For this review, take the finished solid that the model builds, in its own axes (mm). A direction names the side the tool comes from. Round coordinates to 2 decimals unless told otherwise and drop trailing zeros. Loops run counter-clockwise (first coordinate to the right, second up) from the corner with the lowest first, then second, coordinate; pieces in that order, holes last. Notation, with made-up numbers: (19, 29.25) -> (51, 29.25) arc R19 ccw to (51, 44.25) -> close; hole circle Ø3 at (65, -24). An arc over 180 degrees is marked (long way). Write each question's results on one line, items separated by ' | '.
```python
from build123d import *

# Parameters (mm, degrees)
SKETCH1_W           = 48
SKETCH1_H           = 48
SKETCH1_W_2         = 40
SKETCH1_H_2         = 40
BOSS_EXTRUDE1_DEPTH = 24
SKETCH1_5_W         = 40
SKETCH1_5_H         = 40
BOSS_EXTRUDE2_DEPTH = 4
SKETCH3_W           = 30
SKETCH3_H           = 30
BOSS_EXTRUDE3_DEPTH = 7
SKETCH4_R           = 2
CUT_EXTRUDE1_DEPTH  = 25


with BuildPart() as part:
    # Sketch1 → Boss-Extrude1 (new body)
    with BuildSketch(Plane(origin=(0, 0, 0), x_dir=(1, 0, 0), z_dir=(0, 1, 0))):
        Rectangle(SKETCH1_W, SKETCH1_H)
        Rectangle(SKETCH1_W_2, SKETCH1_H_2, mode=Mode.SUBTRACT)
    extrude(amount=BOSS_EXTRUDE1_DEPTH)

    # Sketch1<5> → Boss-Extrude2 (add)
    with BuildSketch(Plane(origin=(0, 0, 0), x_dir=(1, 0, 0), z_dir=(0, 1, 0))):
        Rectangle(SKETCH1_5_W, SKETCH1_5_H)
    extrude(amount=BOSS_EXTRUDE2_DEPTH)

    # Sketch3 → Boss-Extrude3 (add)
    with BuildSketch(Plane(origin=(0, 4, 0), x_dir=(1, 0, 0), z_dir=(0, 1, 0))):
        Rectangle(SKETCH3_W, SKETCH3_H)
    extrude(amount=BOSS_EXTRUDE3_DEPTH)

    # Sketch4 → Cut-Extrude1 (cut)
    with BuildSketch(Plane(origin=(24, 0, 0), x_dir=(0, 0, -1), z_dir=(1, 0, 0))):
        with Locations((10, 7.5)):
            Circle(SKETCH4_R)
    extrude(amount=-CUT_EXTRUDE1_DEPTH, mode=Mode.SUBTRACT)


solid = part.part
```
1. Consider section A-A (y = 22.25). State the section outline as (x, z) points.
Values found:
outline: (-24, -24) -> (24, -24) -> (24, 24) -> (-24, 24) -> close; hole (-20, -20) -> (20, -20) -> (20, 20) -> (-20, 20) -> close
2. To check wall thickness, follow probe 1 along Z at (x, y) = (-13, 7.5); probe 2 along Y at (x, z) = (10, -10). State the ranges of each line that lie inside material, in increasing order.
Values found:
probe 1: z = -24 to -20, -15 to 15, 20 to 24 | probe 2: y = 0 to 5.5, 9.5 to 11
3. Consider section C-C (z = -10). State the section outline as (x, y) points, plus the area to 3 significant figures.
Values found:
outline: (-24, 0) -> (24, 0) -> (24, 5.5) -> (20, 5.5) -> (20, 4) -> (15, 4) -> (15, 5.5) -> (-1, 5.5) -> (-1, 9.5) -> (15, 9.5) -> (15, 11) -> (-15, 11) -> (-15, 4) -> (-20, 4) -> (-20, 24) -> (-24, 24) -> close; (20, 9.5) -> (24, 9.5) -> (24, 24) -> (20, 24) -> close | area: 482 mm2
4. For pin 1 (15 mm diameter, centred on x = -7, z = 5.5, fed in from +Y), flat-tipped, find the tip position at first contact; note if it passes through.
Values found:
pin 1: stops at y = 11
5. Draft analysis for pull direction X (two halves, no side actions). For faces 4 (the face through (0, 0, 0)), 5 (the face through (0, 7, 15)), 6 (the face through (24, 12, 0)), state which applies: released by +X, released by -X, zero draft, split by the parting line, or undercut.
Values found:
face 4: zero draft | face 5: undercut | face 6: released by +X
6. Tool access review of faces 1 (the face through (0, 7, -15)), 2 (the face through (-1, 8, -10)), 3 (the face through (21, 24, 0)): name each direction out of +Z, -Z, +X, -X, +Y, -Y from which nothing blocks a thin tool from reaching the whole face with its end or side.
Values found:
face 1: +Y | face 2: +X | face 3: +Z, -Z, +X, -X, +Y
7. Consider section B-B (x = -4.5). State the section outline as (y, z) points, plus the area to 3 significant figures.
Values found:
outline: (0, -24) -> (24, -24) -> (24, -20) -> (4, -20) -> (4, -15) -> (11, -15) -> (11, 15) -> (4, 15) -> (4, 20) -> (24, 20) -> (24, 24) -> (0, 24) -> close | area: 562 mm2
8. Consider section D-D (y = 7.5). State the section outline as (x, z) points, plus the area to 3 significant figures.
Values found:
outline: (-24, -24) -> (24, -24) -> (24, -12) -> (20, -12) -> (20, -20) -> (-20, -20) -> (-20, 20) -> (20, 20) -> (20, -8) -> (24, -8) -> (24, 24) -> (-24, 24) -> close; (-15, -15) -> (15, -15) -> (15, -12) -> (-1, -12) -> (-1, -8) -> (15, -8) -> (15, 15) -> (-15, 15) -> close | area: 1,520 mm2
